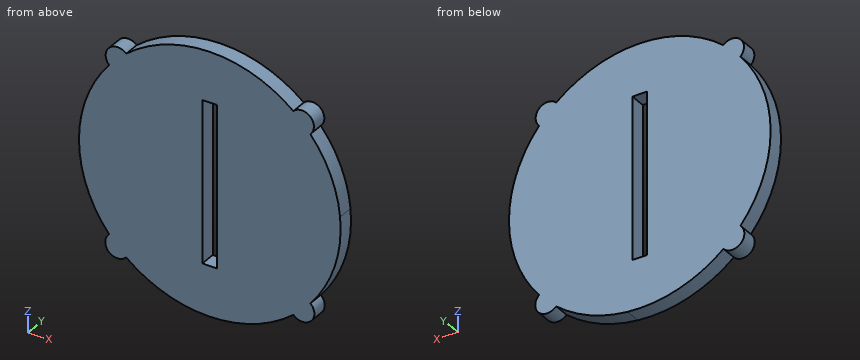
from build123d import *

# Parameters (mm, degrees)
BOSS_EXTRUDE1_DEPTH = 4


with BuildPart() as part:
    # Sketch1 → Boss-Extrude1 (new body)
    with BuildSketch(Plane(origin=(0, 0, 0), x_dir=(1, 0, 0), z_dir=(0, 1, 0))):
        with BuildLine():
            ThreePointArc((-71.868882923, 41.744528782), (-71.873310505, 41.73919705), (-71.877736955, 41.733864379))
            ThreePointArc((-71.877736955, 41.733864379), (-79.402730452, 20.871324191), (-71.862759828, 0.01419224))
            ThreePointArc((-71.862759828, 0.01419224), (-71.861231345, -4.243487526), (-67.603551579, -4.241959043))
            ThreePointArc((-67.603551579, -4.241959043), (-46.752732556, -11.766954644), (-25.901913533, -4.241959043))
            ThreePointArc((-25.901913533, -4.241959043), (-21.644233766, -4.243487526), (-21.642705283, 0.01419224))
            ThreePointArc((-21.642705283, 0.01419224), (-16.577915273, 8.412965085), (-14.235919977, 17.936963257))
            ThreePointArc((-14.235919977, 17.936963257), (-15.574380313, 30.574941531), (-21.636582188, 41.744528782))
            ThreePointArc((-21.636582188, 41.744528782), (-21.535327773, 46.082350824), (-25.873221397, 45.984210943))
            ThreePointArc((-25.873221397, 45.984210943), (-34.22276847, 51.033045356), (-43.691357182, 53.389206016))
            ThreePointArc((-43.691357182, 53.389206016), (-56.400529129, 52.075071922), (-67.632243714, 45.984210943))
            ThreePointArc((-67.632243714, 45.984210943), (-71.970137338, 46.082350824), (-71.868882923, 41.744528782))
        make_face()
        Polygon((-48.602732556, 0.733045356), (-48.602732556, 20.883045356), (-48.602732556, 41.033045356), (-44.902732556, 41.033045356), (-44.902732556, 20.883045356), (-44.902732556, 0.733045356), align=None, mode=Mode.SUBTRACT)
    extrude(amount=BOSS_EXTRUDE1_DEPTH)


solid = part.part
CAD build for the part. Positions are in the model's coordinates, mm. Round coordinates to 2 decimals unless told otherwise and drop trailing zeros. Order: outer loops, then holes, each group sorted by start corner. A loop starts at its lowest first (then second) coordinate and runs counter-clockwise, first axis right, second up. Notation, with made-up numbers: (85, -27) -> (95, -27) arc R23 ccw to (95, 7) -> close; hole circle Ø9 at (14.25, 8). An arc over 180 degrees is marked (long way). Write each question's results on one line, items separated by ' | '.
1. Flat gauge pins, fed straight in: P1, Ø1.5, axis at x = -62.5, y = 2, coming from the +Z side; P2, Ø1.1, axis at x = -47, y = 1, coming from the +Z side; P3, Ø1.2, axis at y = 3, z = -11, coming from the -X side. Where does each tip first touch, or does it go through?
Findings below:
P1: stops at z = 8.12 | P2: stops at z = 11.77 | P3: stops at x = -78.06
2. Cut at C-C (z = -16). Give the cut face in (x, y).
Findings below:
outline: (-79.04, 0) -> (-48.6, 0) -> (-48.6, 4) -> (-79.04, 4) -> close; (-44.9, 0) -> (-14.47, 0) -> (-14.47, 4) -> (-44.9, 4) -> close
3. Cut at D-D (x = -70). Give the cut face in (y, z).
Findings below:
outline: (0, -46.96) -> (4, -46.96) -> (4, 5.11) -> (0, 5.11) -> close
4. Cut at B-B (z = -31). Give the cut face in (x, y).
Findings below:
outline: (-77.8, 0) -> (-48.6, 0) -> (-48.6, 4) -> (-77.8, 4) -> close; (-44.9, 0) -> (-15.71, 0) -> (-15.71, 4) -> (-44.9, 4) -> close
5. Wall check: line 1 along X through (y, z) = (0.35, -20); line 2 along Z through (x, y) = (-21, 1.65); line 3 along Z through (x, y) = (-47, 2.85). Give the ranges that are in metal, low to high. Write a range as [from, to].
Findings below:
line 1: x = [-79.39, -48.6], [-44.9, -14.11] | line 2: z = [-45.35, -42.57], [-40.95, -0.81], [0.94, 3.29] | line 3: z = [-53.53, -41.03], [-0.73, 11.77]
